Can you work these out from the model? Positions are in its coordinate system, mm. A direction names the side the tool comes from. Give positions to 0.01 mm unless a question says otherwise; leave off trailing zeros. Write each loop counter-clockwise with the first axis right and the second up, starting at its lowest first coordinate (ties: lowest second). Pieces come first, ordered by that corner, then holes.
1. If I drill on probe 1 along X at (y, z) = (0.95, 5.75); probe 2 along Y at (x, z) = (3.75, 8), over which ranges is the centre line in solid material (lowest first)?
2. On a 3-axis mill with a long thin cutter (end or side, diameter ignored), from which of +Z, -Z, +X, -X, +Y, -Y can I reach the whole of each face in a straight line? I mean faces 1 (the flat face through (-4, 4, 0)), 2 (the flat face through (4, 4, 0)), 3 (the flat face through (0, 4, 15)). Say none if no direction works.
3. Suppose I cut it at B-B (y = 3.7). Please give me the cut outline in (x, z).
4. Suppose I cut it at C-C (x = 5.25). Please give me the cut outline in (y, z), and give its area (3 significant figures).
5. I'm going to push flat-ended pins straight in: pin 1 (2 mm diameter, centred on x = -4, z = 6, fed in from -Y); pin 2 (3 mm diameter, centred on y = 2, z = -7, fed in from -X). Where does each tip first touch, or does it pass through?
6. Suppose I cut it at A-A (z = -3.25). Please give me the cut outline in (x, y), and give its area (3 significant figures).
```python
from build123d import *

# Parameters (mm, degrees)
F0_W     = 2
F0_H     = 2
F0_W_2   = 4
F1_DEPTH = 15


with BuildPart() as f1:
    # F0 (on Top) → F1 (new body, symmetric)
    with BuildSketch(Plane.XY):
        with Locations((-1, 5)):
            Rectangle(F0_W, F0_H)
        with Locations((1, 5)):
            Rectangle(F0_W, F0_H)
        with Locations((4, 5)):
            Rectangle(F0_W_2, F0_H)
        Polygon((-2, 4), (-2, 0), (2, 0), (2, 4), (0, 4), align=None)
        with Locations((-4, 5)):
            Rectangle(F0_W_2, F0_H)
    extrude(amount=F1_DEPTH, both=True)


solid = f1.part
```
Checks:
1. probe 1: x = -2 to 2
1. probe 2: y = 4 to 6
2. face 1: +Z, -Z, -X, -Y
2. face 2: +Z, -Z, +X, -Y
2. face 3: +Z, +X, -X, +Y, -Y
3. outline: (-2, -15) - (2, -15) - (2, 15) - (-2, 15) - close
4. outline: (4, -15) - (6, -15) - (6, 15) - (4, 15) - close
4. area: 60.0 mm2
5. pin 1: stops at y = 4
5. pin 2: stops at x = -2
6. outline: (-6, 4) - (-2, 4) - (-2, 0) - (2, 0) - (2, 4) - (6, 4) - (6, 6) - (-6, 6) - close
6. area: 40.0 mm2
